```python
from build123d import *

# Parameters (mm, degrees)
SKETCH_1_W      = 16
SKETCH_1_H      = 16
EXTRUDE_1_DEPTH = 3
SKETCH_2_W      = 18
SKETCH_2_H      = 18
EXTRUDE_2_DEPTH = 1


with BuildPart() as part:
    # Эскиз1 → Бобышка-Вытянуть1 (new, symmetric)
    with BuildSketch(Plane(origin=(0, 0, 0), x_dir=(1, 0, 0), z_dir=(0, 1, 0))):
        Rectangle(SKETCH_1_W, SKETCH_1_H)
    extrude(amount=EXTRUDE_1_DEPTH, both=True)

    # Эскиз2 → Бобышка-Вытянуть2 (add)
    with BuildSketch(Plane(origin=(0, 3, 0), x_dir=(1, 0, 0), z_dir=(0, 1, 0))):
        Rectangle(SKETCH_2_W, SKETCH_2_H)
    extrude_2 = extrude(amount=EXTRUDE_2_DEPTH)

    # Зеркальное отражение1: Бобышка-Вытянуть2 across plane
    add(extrude_2.mirror(Plane.ZX))


solid = part.part
```
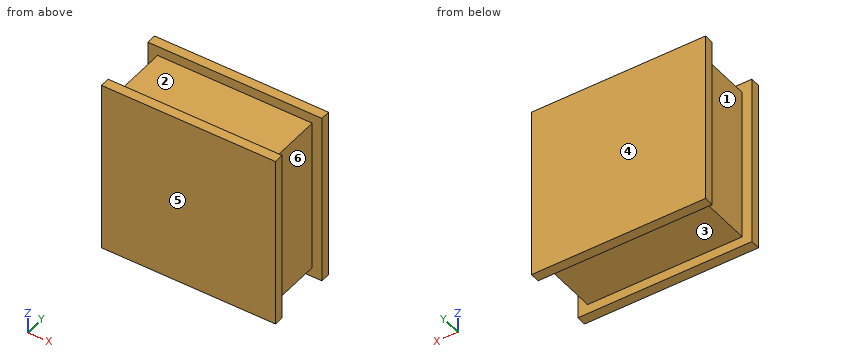
Can you work these out from the model? Positions are in its coordinate system, mm. Face numbers are marked on the shaded views. A direction names the side the tool comes from. Coordinates: 2 decimals unless noted, no trailing zeros. Loops run counter-clockwise (first coordinate to the right, second up) from the corner with the lowest first, then second, coordinate; pieces in that order, holes last.
1) Thinking about a two-plate mould opening in Y: for the marked faces 4, 5 and 6, which applies, pulls with the +Y half, pulls with the -Y half, needs draft (parallel to the pull), parting line crosses it, or undercut?
2) Imagine slicing it at B-B on x = 4. List the corners of the cut face in (y, z) for me, plus the area to 3 significant figures.
3) For pin 1 (2 mm diameter, centred on y = 0.5, z = -1, fed in from +X); pin 2 (1.8 mm diameter, centred on x = 2.5, y = 1, fed in from -Z); pin 3 (4 mm diameter, centred on x = -0.5, y = 0, fed in from +Z), each with a flat end and sliding along its axis, tell me the tip position at first contact or that it passes through.
4) Imagine slicing it at C-C on y = 0. List the corners of the cut face in (x, z) for me.
5) Which directions (+Z, -Z, +X, -X, +Y, -Y) give clear straight access to the entire face, cutting with the end or side of a thin tool? Please do the marked faces 1, 2 and 3.
6) Imagine slicing it at A-A on z = 0.75. List the corners of the cut face in (x, y) for me.
7) I need wall thicknesses on probe 1 along Z at (x, y) = (1, 0.5). Which ranges of the line are inside material? Lowest first, please.
Completed:
1. face 4: pulls with the +Y half
1. face 5: pulls with the -Y half
1. face 6: undercut
2. outline: (-4, -9) - (-3, -9) - (-3, -8) - (3, -8) - (3, -9) - (4, -9) - (4, 9) - (3, 9) - (3, 8) - (-3, 8) - (-3, 9) - (-4, 9) - close
2. area: 132 mm2
3. pin 1: stops at x = 8
3. pin 2: stops at z = -8
3. pin 3: stops at z = 8
4. outline: (-8, -8) - (8, -8) - (8, 8) - (-8, 8) - close
5. face 1: +Z, -Z, -X
5. face 2: +Z, +X, -X
5. face 3: -Z, +X, -X
6. outline: (-9, -4) - (9, -4) - (9, -3) - (8, -3) - (8, 3) - (9, 3) - (9, 4) - (-9, 4) - (-9, 3) - (-8, 3) - (-8, -3) - (-9, -3) - close
7. probe 1: z = -8 to 8
